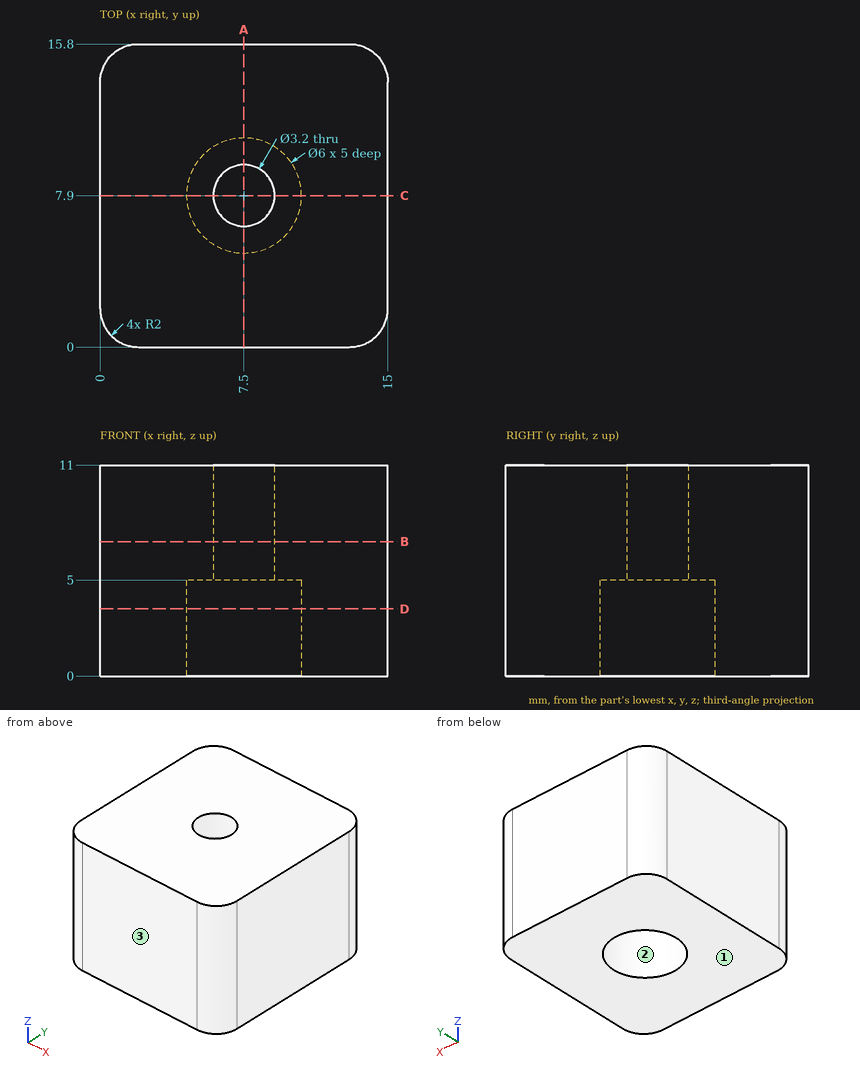
Geometry: see drawing. Coordinates: mm, zero at the bounding-box minimum. Give positions to 0.01 mm unless a question says otherwise; leave off trailing zeros. Write each loop counter-clockwise with the first axis right and the second up, starting at its lowest first coordinate (ties: lowest second). Pieces come first, ordered by that corner, then holes. Notation, with made-up numbers: M 46,-20.5 L 58,-20.5 A31 ccw 58,7.5 Z; hole C 63.25,-12.75 d5. An arc over 180 degrees is marked long. Answer as a JSON object with one key per item and string values.
Q1. Mould query, pull axis Y, two halves, no side actions, for the marked faces 1, 2 and 3. Classes: +Y half, -Y half, draft (parallel to the pull), parting line (faces both ways), or undercut.
Geometry check:
{"face 1": "draft", "face 2": "undercut", "face 3": "-Y half"}
Q2. Contact query for a flat-ended pin moving along its axis: P1, Ø1.9, axis at x = 7.5, y = 7.9, coming from the +Z side. Output: stop coordinate, or through.
Geometry check:
{"P1": "passes through"}
Q3. Cut plane C-C, the plane y = 7.9. Return the cut outline in (x, z), then the cut area to 3 significant figures.
Geometry check:
{"outline": "M 0,0 L 4.5,0 L 4.5,5 L 5.9,5 L 5.9,11 L 0,11 Z; M 9.1,5 L 10.5,5 L 10.5,0 L 15,0 L 15,11 L 9.1,11 Z", "area": "116 mm^2"}
Q4. Ray query, line 1 along Y through (x, z) = (7.5, 3.55); line 2 along Y through (x, z) = (7.5, 7.1); line 3 along Z through (x, y) = (9.25, 9.5). Return the intervals inside material, ascending.
Geometry check:
{"line 1": "y = 0 to 4.9, 10.9 to 15.8", "line 2": "y = 0 to 6.3, 9.5 to 15.8", "line 3": "z = 5 to 11"}
Q5. Cut plane A-A, the plane x = 7.5. Return the cut outline in (y, z), then the cut area to 3 significant figures.
Geometry check:
{"outline": "M 0,0 L 4.9,0 L 4.9,5 L 6.3,5 L 6.3,11 L 0,11 Z; M 9.5,5 L 10.9,5 L 10.9,0 L 15.8,0 L 15.8,11 L 9.5,11 Z", "area": "125 mm^2"}
Q6. Cut plane B-B, the plane z = 7. Return the cut outline in (x, y).
Geometry check:
{"outline": "M 0,2 A2 ccw 2,0 L 13,0 A2 ccw 15,2 L 15,13.8 A2 ccw 13,15.8 L 2,15.8 A2 ccw 0,13.8 Z; hole C 7.5,7.9 d3.2"}
Q7. Cut plane D-D, the plane z = 3.5. Return the cut outline in (x, y), then the cut area to 3 significant figures.
Geometry check:
{"outline": "M 0,2 A2 ccw 2,0 L 13,0 A2 ccw 15,2 L 15,13.8 A2 ccw 13,15.8 L 2,15.8 A2 ccw 0,13.8 Z; hole C 7.5,7.9 d6", "area": "205 mm^2"}
